For this review, take the finished solid that the model builds, in its own axes (mm). A direction names the side the tool comes from. Round coordinates to 2 decimals unless told otherwise and drop trailing zeros. Order: outer loops, then holes, each group sorted by start corner. A loop starts at its lowest first (then second) coordinate and runs counter-clockwise, first axis right, second up. Notation, with made-up numbers: (-18.5, 32.25) - (6.5, 32.25) arc R22 ccw to (6.5, 57.25) - close; hole circle Ø8 at (32, 42). An arc over 180 degrees is marked (long way). One line per item, written item: value.
```python
from build123d import *

# Parameters (mm, degrees)
F1_DEPTH  = 2.8
F0_W      = 62.5
F0_H      = 36
F2_DEPTH  = 9
F3_W      = 36
F3_H      = 1.5
F4_DEPTH  = 62.5
F5_R      = 2.5
F6_DEPTH  = 1
F9_W      = 20.4
F9_H      = 15.6
F10_DEPTH = 13.301
F12_DEPTH = 50


# Not quite as in the source:
# - a feature names something its author has since deleted; it is built from what else it names


with BuildPart() as f1:
    # F0 (on Top) → F1 (new body)
    with BuildSketch(Plane.XY):
        Polygon((29.8387005084, 17), (-30.1612994916, 17), (-30.1612994916, -17), (29.8387005084, -17), (29.8387005084, -15.5), (-28.6612994916, -15.5), (-28.6612994916, 15.5), (29.8387005084, 15.5), align=None)
    extrude(amount=-F1_DEPTH)

    # F0 (on Top) → F2 (join)
    with BuildSketch(Plane.XY):
        with Locations((0.0887005084, 0)):
            Rectangle(F0_W, F0_H)
        Polygon((-30.1612994916, -17), (-30.1612994916, 17), (29.8387005084, 17), (29.8387005084, 15.5), (29.8387005084, -15.5), (29.8387005084, -17), align=None, mode=Mode.SUBTRACT)
        Polygon((29.8387005084, 17), (-30.1612994916, 17), (-30.1612994916, -17), (29.8387005084, -17), (29.8387005084, -15.5), (-28.6612994916, -15.5), (-28.6612994916, 15.5), (29.8387005084, 15.5), align=None)
    extrude(amount=F2_DEPTH)

    # F3 (on face) → F4 (join, through all)
    with BuildSketch(Plane.YZ.offset(31.3387005084)):
        with Locations((0, 9.75)):
            Rectangle(F3_W, F3_H)
    extrude(amount=-F4_DEPTH)

    # F5
    f5_edges = [f1.edges().sort_by_distance(p)[0] for p in [
        (31.338701, 0, 10.5),
        (0.088701, -18, 10.5),
        (31.338701, -18, 5.25),
        (31.338701, 18, 5.25),
        (0.088701, 18, 10.5),
        (-31.161299, 18, 5.25),
        (-31.161299, 0, 10.5),
        (-31.161299, -18, 5.25),
    ]]
    fillet(f5_edges, radius=F5_R)

    # F6 (cut): a face of the model
    f6_faces = [f1.faces().sort_by_distance(p)[0] for p in [
        (-28.6612994916, 0, 3.1),
    ]]
    extrude(f6_faces, amount=-F6_DEPTH, mode=Mode.SUBTRACT)

    # F9 (on face) → F10 (cut, through all)
    with BuildSketch(Plane.XY.offset(10.5)):
        with Locations((-10.4612994916, 0)):
            Rectangle(F9_W, F9_H)
    extrude(amount=-F10_DEPTH, mode=Mode.SUBTRACT)

    # F11 (on face) → F12 (cut)
    with BuildSketch(Plane.XZ.offset(18)):
        Polygon((-23.7249415368, 7.122464478), (-25.6706383079, 1.9621371757), (-24.4017057121, 1.9621371757), (-22.4560089409, 7.122464478), align=None)
        Polygon((-15.7249415368, 7.122464478), (-17.6706383079, 1.9621371757), (-16.4017057121, 1.9621371757), (-14.4560089409, 7.122464478), align=None)
        Polygon((-7.7249415368, 7.122464478), (-9.6706383079, 1.9621371757), (-8.4017057121, 1.9621371757), (-6.4560089409, 7.122464478), align=None)
        Polygon((0.2750584632, 7.122464478), (-1.6706383079, 1.9621371757), (-0.4017057121, 1.9621371757), (1.5439910591, 7.122464478), align=None)
        Polygon((8.2750584632, 7.122464478), (6.3293616921, 1.9621371757), (7.5982942879, 1.9621371757), (9.5439910591, 7.122464478), align=None)
        Polygon((16.2750584632, 7.122464478), (14.3293616921, 1.9621371757), (15.5982942879, 1.9621371757), (17.5439910591, 7.122464478), align=None)
        Polygon((24.2750584632, 7.122464478), (22.3293616921, 1.9621371757), (23.5982942879, 1.9621371757), (25.5439910591, 7.122464478), align=None)
    extrude(amount=-F12_DEPTH, mode=Mode.SUBTRACT)


solid = f1.part
```
Item 1: Machinability: for faces 1 (the flat face through (1, 0, 9)), 2 (the flat face through (-16.684, 16.732, 4.578)), 3 (the flat face through (-11, 7.8, 10)), which of the approach directions +Z, -Z, +X, -X, +Y, -Y give a long, thin tool a straight path to every point of the face, cutting with its end or side? Answer none if there is none.
Returned:
face 1: -Z
face 2: +Y, -Y
face 3: +Z, -Z
Item 2: For P1, Ø1.4, axis at y = 4.5, z = -1, coming from the -X side; P2, Ø0.6, axis at x = -1, y = -16.5, coming from the +Z side; P3, Ø1.4, axis at x = -12, z = -1.5, coming from the +Y side, all flat-tipped, find the tip position at first contact; note any pin that passes through.
Returned:
P1: x = -30.16
P2: z = 10.4
P3: y = 17
Item 3: Take a section at A-A (y = 4.5). Write out the cut boundary in (x, z).
Returned:
outline: (-31.16, 0) - (-30.16, 0) - (-30.16, -2.8) - (-29.66, -2.8) - (-29.66, 9) - (-20.66, 9) - (-20.66, 10.5) - (-28.66, 10.5) arc R2.5 ccw to (-31.16, 8) - close; (-0.26, 9) - (29.84, 9) - (29.84, 0) - (31.34, 0) - (31.34, 8) arc R2.5 ccw to (28.84, 10.5) - (-0.26, 10.5) - close
Item 4: Take a section at C-C (x = 23). Write out the cut boundary in (y, z), plus the area to 3 significant figures.
Returned:
outline: (-18, 0) - (-17, 0) - (-17, -2.8) - (-15.5, -2.8) - (-15.5, 1.96) - (-18, 1.96) - close; (-18, 3.74) - (-15.5, 3.74) - (-15.5, 9) - (15.5, 9) - (15.5, 3.74) - (18, 3.74) - (18, 8) arc R2.5 ccw to (15.5, 10.5) - (-15.5, 10.5) arc R2.5 ccw to (-18, 8) - close; (15.5, -2.8) - (17, -2.8) - (17, 0) - (18, 0) - (18, 1.96) - (15.5, 1.96) - close
area: 95.8 mm^2
Item 5: Take a section at D-D (z = -1.25). Write out the cut boundary in (x, y), plus the area to 4 significant figures.
Returned:
outline: (-30.16, -17) - (29.84, -17) - (29.84, -15.5) - (-29.66, -15.5) - (-29.66, 15.5) - (29.84, 15.5) - (29.84, 17) - (-30.16, 17) - close
area: 195.5 mm^2
Item 6: The part is to be moulded in two halves that separate along Z. For faces 4 (the flat face through (-30.161, 0, -1)), 5 (the flat face through (-16.684, -16.768, 4.578)), 6 (the flat face through (0, 0, 10.5)), 7 (the flat face through (-0.684, -16.768, 4.578)), say which applies: +Z half, -Z half, draft (parallel to the pull), parting line (faces both ways), or undercut.
Returned:
face 4: draft
face 5: undercut
face 6: +Z half
face 7: undercut
Item 7: Take a section at B-B (y = 12.5). Write out the cut boundary in (x, z), plus the area to 3 significant figures.
Returned:
outline: (-31.16, 0) - (-30.16, 0) - (-30.16, -2.8) - (-29.66, -2.8) - (-29.66, 9) - (29.84, 9) - (29.84, 0) - (31.34, 0) - (31.34, 8) arc R2.5 ccw to (28.84, 10.5) - (-28.66, 10.5) arc R2.5 ccw to (-31.16, 8) - close
area: 119 mm^2
Item 8: Wall thickness on line 1 (Y direction, x = 23.5, z = 0.5); line 2 (X direction, y = 10.5, z = 5.5); line 3 (Y direction, x = 4, z = -1): over which ranges is each line inside the solid? List them lowest first.
Returned:
line 1: -18 to -15.5, 15.5 to 18
line 2: -31.16 to -29.66, 29.84 to 31.34
line 3: -17 to -15.5, 15.5 to 17
